from build123d import *

# Parameters (mm, degrees)
BOSS_EXTRUDE1_START  = 77.2
SKETCH1_R            = 13.2
BOSS_EXTRUDE1_DEPTH  = 8
BOSS_EXTRUDE2_START  = 79.9
SKETCH2_R            = 20
BOSS_EXTRUDE2_DEPTH  = 2.6
BOSS_EXTRUDE3_START  = 79.9
SKETCH3_R            = 11.75
BOSS_EXTRUDE3_DEPTH  = 2.6
BOSS_EXTRUDE4_START  = 76.7
SKETCH4_R            = 4.6
BOSS_EXTRUDE4_DEPTH  = 2.3
BOSS_EXTRUDE5_START  = -55.3
SKETCH5_W            = 2.3
SKETCH5_H            = 11.5
BOSS_EXTRUDE5_DEPTH  = 6.6
BOSS_EXTRUDE6_START  = -52.9
SKETCH6_W            = 10
SKETCH6_H            = 4.5
BOSS_EXTRUDE6_DEPTH  = 1.8
BOSS_EXTRUDE7_START  = -55.3
SKETCH7_W            = 2.3
SKETCH7_H            = 11.5
BOSS_EXTRUDE7_DEPTH  = 6.6
BOSS_EXTRUDE8_START  = -52.9
SKETCH8_W            = 10
SKETCH8_H            = 4.5
BOSS_EXTRUDE8_DEPTH  = 1.8
BOSS_EXTRUDE9_START  = -52
SKETCH9_W            = 2.3
SKETCH9_H            = 6.6
BOSS_EXTRUDE9_DEPTH  = 11.5
BOSS_EXTRUDE10_START = -46.5
SKETCH10_W           = 10
SKETCH10_H           = 1.8
BOSS_EXTRUDE10_DEPTH = 4.5
BOSS_EXTRUDE11_START = -63.5
SKETCH11_W           = 2.3
SKETCH11_H           = 6.6
BOSS_EXTRUDE11_DEPTH = 11.5
BOSS_EXTRUDE12_START = -62
SKETCH12_W           = 10
SKETCH12_H           = 1.8
BOSS_EXTRUDE12_DEPTH = 4.5
BOSS_EXTRUDE13_START = 76.2
SKETCH13_R           = 3
BOSS_EXTRUDE13_DEPTH = 10


with BuildPart() as part:
    # Sketch1 → Boss-Extrude1 (new body)
    with BuildSketch(Plane(origin=(0, 0, 0), x_dir=(0, 0, -1), z_dir=(1, 0, 0)).offset(BOSS_EXTRUDE1_START)):
        with Locations((52, -65)):
            Circle(SKETCH1_R)
    extrude(amount=BOSS_EXTRUDE1_DEPTH)


with BuildPart() as body_2:
    # Sketch2 → Boss-Extrude2 (new body)
    with BuildSketch(Plane(origin=(0, 0, 0), x_dir=(0, 0, -1), z_dir=(1, 0, 0)).offset(BOSS_EXTRUDE2_START)):
        with Locations((52, -65)):
            Circle(SKETCH2_R)
    extrude(amount=BOSS_EXTRUDE2_DEPTH)


with BuildPart() as part_1:
    add(part.part)

    # Combine1: cut body 2
    add(body_2.part, mode=Mode.SUBTRACT)

    # Sketch3 → Boss-Extrude3 (add)
    with BuildSketch(Plane(origin=(0, 0, 0), x_dir=(0, 0, -1), z_dir=(1, 0, 0)).offset(BOSS_EXTRUDE3_START)):
        with Locations((52, -65)):
            Circle(SKETCH3_R)
    extrude(amount=BOSS_EXTRUDE3_DEPTH)


with BuildPart() as body_2_2:
    # Sketch4 → Boss-Extrude4 (new body)
    with BuildSketch(Plane(origin=(0, 0, 0), x_dir=(0, 0, -1), z_dir=(1, 0, 0)).offset(BOSS_EXTRUDE4_START)):
        with Locations((52, -65)):
            Circle(SKETCH4_R)
    extrude(amount=BOSS_EXTRUDE4_DEPTH)


with BuildPart() as part_2:
    add(part_1.part)

    # Combine2: cut body 2 2
    add(body_2_2.part, mode=Mode.SUBTRACT)


with BuildPart() as body_2_3:
    # Sketch5 → Boss-Extrude5 (new body)
    with BuildSketch(Plane.XY.offset(BOSS_EXTRUDE5_START)):
        with Locations((77.85, -59.25)):
            Rectangle(SKETCH5_W, SKETCH5_H)
    extrude(amount=BOSS_EXTRUDE5_DEPTH)


with BuildPart() as part_3:
    add(part_2.part)

    # Combine3: cut body 2 3
    add(body_2_3.part, mode=Mode.SUBTRACT)


with BuildPart() as body_2_4:
    # Sketch6 → Boss-Extrude6 (new body)
    with BuildSketch(Plane.XY.offset(BOSS_EXTRUDE6_START)):
        with Locations((81.2, -57.25)):
            Rectangle(SKETCH6_W, SKETCH6_H)
    extrude(amount=BOSS_EXTRUDE6_DEPTH)


with BuildPart() as part_4:
    add(part_3.part)

    # Combine4: cut body 2 4
    add(body_2_4.part, mode=Mode.SUBTRACT)


with BuildPart() as body_2_5:
    # Sketch7 → Boss-Extrude7 (new body)
    with BuildSketch(Plane.XY.offset(BOSS_EXTRUDE7_START)):
        with Locations((77.85, -70.75)):
            Rectangle(SKETCH7_W, SKETCH7_H)
    extrude(amount=BOSS_EXTRUDE7_DEPTH)


with BuildPart() as part_5:
    add(part_4.part)

    # Combine5: cut body 2 5
    add(body_2_5.part, mode=Mode.SUBTRACT)


with BuildPart() as body_2_6:
    # Sketch8 → Boss-Extrude8 (new body)
    with BuildSketch(Plane.XY.offset(BOSS_EXTRUDE8_START)):
        with Locations((81.2, -72.75)):
            Rectangle(SKETCH8_W, SKETCH8_H)
    extrude(amount=BOSS_EXTRUDE8_DEPTH)


with BuildPart() as part_6:
    add(part_5.part)

    # Combine6: cut body 2 6
    add(body_2_6.part, mode=Mode.SUBTRACT)


with BuildPart() as body_2_7:
    # Sketch9 → Boss-Extrude9 (new body)
    with BuildSketch(Plane.XY.offset(BOSS_EXTRUDE9_START)):
        with Locations((77.85, -65)):
            Rectangle(SKETCH9_W, SKETCH9_H)
    extrude(amount=BOSS_EXTRUDE9_DEPTH)


with BuildPart() as part_7:
    add(part_6.part)

    # Combine7: cut body 2 7
    add(body_2_7.part, mode=Mode.SUBTRACT)


with BuildPart() as body_2_8:
    # Sketch10 → Boss-Extrude10 (new body)
    with BuildSketch(Plane.XY.offset(BOSS_EXTRUDE10_START)):
        with Locations((81.2, -65)):
            Rectangle(SKETCH10_W, SKETCH10_H)
    extrude(amount=BOSS_EXTRUDE10_DEPTH)


with BuildPart() as part_8:
    add(part_7.part)

    # Combine8: cut body 2 8
    add(body_2_8.part, mode=Mode.SUBTRACT)


with BuildPart() as body_2_9:
    # Sketch11 → Boss-Extrude11 (new body)
    with BuildSketch(Plane.XY.offset(BOSS_EXTRUDE11_START)):
        with Locations((77.85, -65)):
            Rectangle(SKETCH11_W, SKETCH11_H)
    extrude(amount=BOSS_EXTRUDE11_DEPTH)


with BuildPart() as part_9:
    add(part_8.part)

    # Combine9: cut body 2 9
    add(body_2_9.part, mode=Mode.SUBTRACT)


with BuildPart() as body_2_10:
    # Sketch12 → Boss-Extrude12 (new body)
    with BuildSketch(Plane.XY.offset(BOSS_EXTRUDE12_START)):
        with Locations((81.2, -65)):
            Rectangle(SKETCH12_W, SKETCH12_H)
    extrude(amount=BOSS_EXTRUDE12_DEPTH)


with BuildPart() as part_10:
    add(part_9.part)

    # Combine10: cut body 2 10
    add(body_2_10.part, mode=Mode.SUBTRACT)


with BuildPart() as body_2_11:
    # Sketch13 → Boss-Extrude13 (new body)
    with BuildSketch(Plane(origin=(0, 0, 0), x_dir=(0, 0, -1), z_dir=(1, 0, 0)).offset(BOSS_EXTRUDE13_START)):
        with Locations((52, -65)):
            Circle(SKETCH13_R)
    extrude(amount=BOSS_EXTRUDE13_DEPTH)


with BuildPart() as part_11:
    add(part_10.part)

    # Combine11: cut body 2 11
    add(body_2_11.part, mode=Mode.SUBTRACT)


solid = part_11.part
Check sheet for the modelled part. Datum: model origin and axes. Units: mm. A direction names the side the tool comes from. Coordinates: 2 decimals unless noted, no trailing zeros. Write each loop counter-clockwise with the first axis right and the second up, starting at its lowest first coordinate (ties: lowest second). Pieces come first, ordered by that corner, then holes.
Item 1: Cross-section at B-B on y = -65. Record the boundary of the cut face in (x, z), then the cut area to 3 significant figures.
Numbers:
outline: (77.2, -65.2) - (79.9, -65.2) - (79.9, -63.75) - (82.5, -63.75) - (82.5, -65.2) - (85.2, -65.2) - (85.2, -62) - (79, -62) - (79, -63.5) - (77.2, -63.5) - close; (77.2, -40.5) - (79, -40.5) - (79, -42) - (85.2, -42) - (85.2, -38.8) - (82.5, -38.8) - (82.5, -40.25) - (79.9, -40.25) - (79.9, -38.8) - (77.2, -38.8) - close; (79, -57.5) - (85.2, -57.5) - (85.2, -55) - (79, -55) - close; (79, -49) - (85.2, -49) - (85.2, -46.5) - (79, -46.5) - close
area: 69.3 mm2
Item 2: Cross-section at A-A on x = 81.5. Record the boundary of the cut face in (y, z).
Numbers:
outline: circle Ø23.5 at (-65, -52); hole (-75, -52.9) - (-70.5, -52.9) - (-70.5, -51.1) - (-75, -51.1) - close; hole circle Ø6 at (-65, -52); hole (-65.9, -62) - (-64.1, -62) - (-64.1, -57.5) - (-65.9, -57.5) - close; hole (-65.9, -46.5) - (-64.1, -46.5) - (-64.1, -42) - (-65.9, -42) - close; hole (-59.5, -52.9) - (-55, -52.9) - (-55, -51.1) - (-59.5, -51.1) - close
Item 3: Mould release check, pull along X, two halves, no side actions. Record for faces 1 (the face through (77.2, -71, -58)), 2 (the face through (79.9, -73, -43)), 3 (the face through (81.18, -64.48, -40.26)), 4 (the face through (78, -68.3, -45)): released by +X, released by -X, zero draft, split by the parting line, or undercut.
Numbers:
face 1: released by -X
face 2: undercut
face 3: undercut
face 4: zero draft
Item 4: Scan lines: probe 1 along Y at (x, z) = (83.5, -52); probe 2 along Z at (x, y) = (83.75, -65); probe 3 along Y at (x, z) = (80.5, -52). Record each from-to range of solid material in increasing order.
Numbers:
probe 1: y = -78.2 to -75, -70.5 to -68, -62 to -59.5, -55 to -51.8
probe 2: z = -65.2 to -62, -57.5 to -55, -49 to -46.5, -42 to -38.8
probe 3: y = -76.75 to -75, -70.5 to -68, -62 to -59.5, -55 to -53.25
Item 5: Cross-section at D-D on z = -61.25. Record the boundary of the cut face in (x, y), then the cut area to 3 significant figures.
Numbers:
outline: (77.2, -74.42) - (79.9, -74.42) - (79.9, -72.25) - (82.5, -72.25) - (82.5, -74.42) - (85.2, -74.42) - (85.2, -65.9) - (79, -65.9) - (79, -68.3) - (77.2, -68.3) - close; (77.2, -61.7) - (79, -61.7) - (79, -64.1) - (85.2, -64.1) - (85.2, -55.58) - (82.5, -55.58) - (82.5, -57.75) - (79.9, -57.75) - (79.9, -55.58) - (77.2, -55.58) - close
area: 116 mm2
Item 6: Depth check by flat-ended pin: pin 1 Ø0.5 at (x, y) = (78, -71) entering from +Z; pin 2 Ø3.5 at (x, z) = (82.5, -44) entering from +Y; pin 3 Ø0.5 at (x, z) = (81.5, -51.5) entering from -Y. Enter the tip coordinate at first touch or a pass-through.
Numbers:
pin 1: stops at z = -40.12
pin 2: stops at y = -53.37
pin 3: stops at y = -76.75
Item 7: Access from +Z, -Z, +X, -X, +Y, -Y to the whole of each face (thin tool, end or side, straight path). Record for faces 5 (the face through (82, -55, -52)), 6 (the face through (78, -53.5, -52)).
Numbers:
face 5: +X, -X
face 6: -X
Item 8: Cross-section at C-C on z = -52. Record the boundary of the cut face in (x, y).
Numbers:
outline: (77.2, -78.2) - (79.9, -78.2) - (79.9, -76.75) - (82.5, -76.75) - (82.5, -78.2) - (85.2, -78.2) - (85.2, -75) - (79, -75) - (79, -76.5) - (77.2, -76.5) - close; (77.2, -53.5) - (79, -53.5) - (79, -55) - (85.2, -55) - (85.2, -51.8) - (82.5, -51.8) - (82.5, -53.25) - (79.9, -53.25) - (79.9, -51.8) - (77.2, -51.8) - close; (79, -70.5) - (85.2, -70.5) - (85.2, -68) - (79, -68) - close; (79, -62) - (85.2, -62) - (85.2, -59.5) - (79, -59.5) - close
